from build123d import *

# Parameters (mm, degrees)
PAD_DEPTH       = 3
POCKET_DEPTH    = 1.5
SKETCH003_R     = 1
POCKET001_DEPTH = 3.001
SKETCH004_W     = 10
SKETCH004_H     = 1.5
PAD001_DEPTH    = 6
FILLET_R        = 3


with BuildPart() as part:
    # Sketch → Pad (new body)
    with BuildSketch(Plane.XY):
        with BuildLine():
            Line((0, 0), (64, 0))
            Line((64, 0), (64, -22))
            ThreePointArc((64, -36), (71, -29), (64, -22))
            Line((64, -36), (64, -58))
            Line((64, -58), (0, -58))
            Line((0, -58), (0, 0))
        make_face()
    extrude(amount=PAD_DEPTH)

    # Sketch001 (on Face7 of Pad) → Pocket (cut)
    with BuildSketch(Plane(origin=(0, 0, 0), x_dir=(1, 0, 0), z_dir=(0, 0, -1))):
        with BuildLine():
            ThreePointArc((64, 22), (71, 29), (64, 36))
            Line((64, 36), (64, 22))
        make_face()
    extrude(amount=-POCKET_DEPTH, mode=Mode.SUBTRACT)

    # Sketch003 → Pocket001 (cut, through all)
    with BuildSketch(Plane.XY.offset(3)):
        with Locations((68.5, -29.25)):
            Circle(SKETCH003_R)
    extrude(amount=-POCKET001_DEPTH, mode=Mode.SUBTRACT)

    # Sketch004 (on Face9 of Pocket001) → Pad001 (join)
    with BuildSketch(Plane(origin=(0, 0, 0), x_dir=(0, -1, 0), z_dir=(-1, 0, 0))):
        with Locations((43, 0.25)):
            Rectangle(SKETCH004_W, SKETCH004_H)
        with Locations((15, 0.25)):
            Rectangle(SKETCH004_W, SKETCH004_H)
    extrude(amount=PAD001_DEPTH)

    # Fillet
    fillet_edges = [part.edges().sort_by_distance(p)[0] for p in [
        (-6, -48, 0.25),
        (-6, -38, 0.25),
        (-6, -20, 0.25),
        (-6, -10, 0.25),
    ]]
    fillet(fillet_edges, radius=FILLET_R)


solid = part.part
Build history of the part. All positions in model axes, mm. A direction names the side the tool comes from. Give positions to 0.01 mm unless a question says otherwise; leave off trailing zeros. Order: outer loops, then holes, each group sorted by start corner. A loop starts at its lowest first (then second) coordinate and runs counter-clockwise, first axis right, second up. Notation, with made-up numbers: M 59.5,3 L 98.5,3 A21 cw 98.5,36 Z; hole C 68,76 d7. An arc over 180 degrees is marked long. Use one line per item in the form item = value.
1) Saw through at D-D (x = 39). Give the cut face in (y, z).
Calculated:
outline = M -58,0 L 0,0 L 0,3 L -58,3 Z
2) Two-plate mould, pull along Y, no slides. Class faces 1 (the face through (-5.1, -38.86, 0.26)), 2 (the face through (36, -29, 3)), 3 (the face through (-5.1, -19.14, 0.26)), 4 (the face through (-5.14, -47.1, 0.26)): released by +Y, released by -Y, zero draft, split by the parting line, or undercut.
Calculated:
face_1 = undercut
face_2 = zero draft
face_3 = undercut
face_4 = released by -Y
3) Drop flat-ended pins along their axis: pin 1 (0.8 mm diameter, centred on x = -1.5, z = 0, fed in from +Y); pin 2 (3.5 mm diameter, centred on x = 68.5, y = -26, fed in from -Z); pin 3 (1.8 mm diameter, centred on x = 68.5, y = -29.25, fed in from -Z); pin 4 (1.6 mm diameter, centred on x = -1, z = 0.5, fed in from -Y). Give the stop position or say it passes through.
Calculated:
pin_1 = -10
pin_2 = 1.5
pin_3 = through
pin_4 = -48
4) Saw through at B-B (x = 68.5). Give the cut face in (y, z).
Calculated:
outline = M -34.36,1.5 L -30.25,1.5 L -30.25,3 L -34.36,3 Z; M -28.25,1.5 L -23.64,1.5 L -23.64,3 L -28.25,3 Z
5) Saw through at C-C (y = -47). Give the cut face in (x, z).
Calculated:
outline = M -5.24,-0.5 L 0,-0.5 L 0,0 L 64,0 L 64,3 L 0,3 L 0,1 L -5.24,1 Z
6) Saw through at A-A (y = -29.25). Give the cut face in (x, z), plus the area to 3 significant figures.
Calculated:
outline = M 0,0 L 64,0 L 64,1.5 L 67.5,1.5 L 67.5,3 L 0,3 Z; M 69.5,1.5 L 71,1.5 L 71,3 L 69.5,3 Z
area = 199 mm2
7) Tool access for faces 5 (the face through (-1, -48, 0)), 6 (the face through (64, -29, 1)), 7 (the face through (-3, -43, 1)), 8 (the face through (-1, -38, 0)): list every direction of +Z, -Z, +X, -X, +Y, -Y with a clear straight run to the whole face (end or side of a thin tool).
Calculated:
face_5 = +Z, -Z, -X, -Y
face_6 = -Z, +X
face_7 = +Z, -X, +Y, -Y
face_8 = +Z, -Z, -X
8) Probe probe 1 along X at (y, z) = (-50, 0.8); probe 2 along Y at (x, z) = (68.5, 2.3); probe 3 along Z at (x, y) = (29.5, -31). List the from-to ranges inside material, lowest first.
Calculated:
probe_1 = 0 to 64
probe_2 = -34.36 to -30.25, -28.25 to -23.64
probe_3 = 0 to 3
